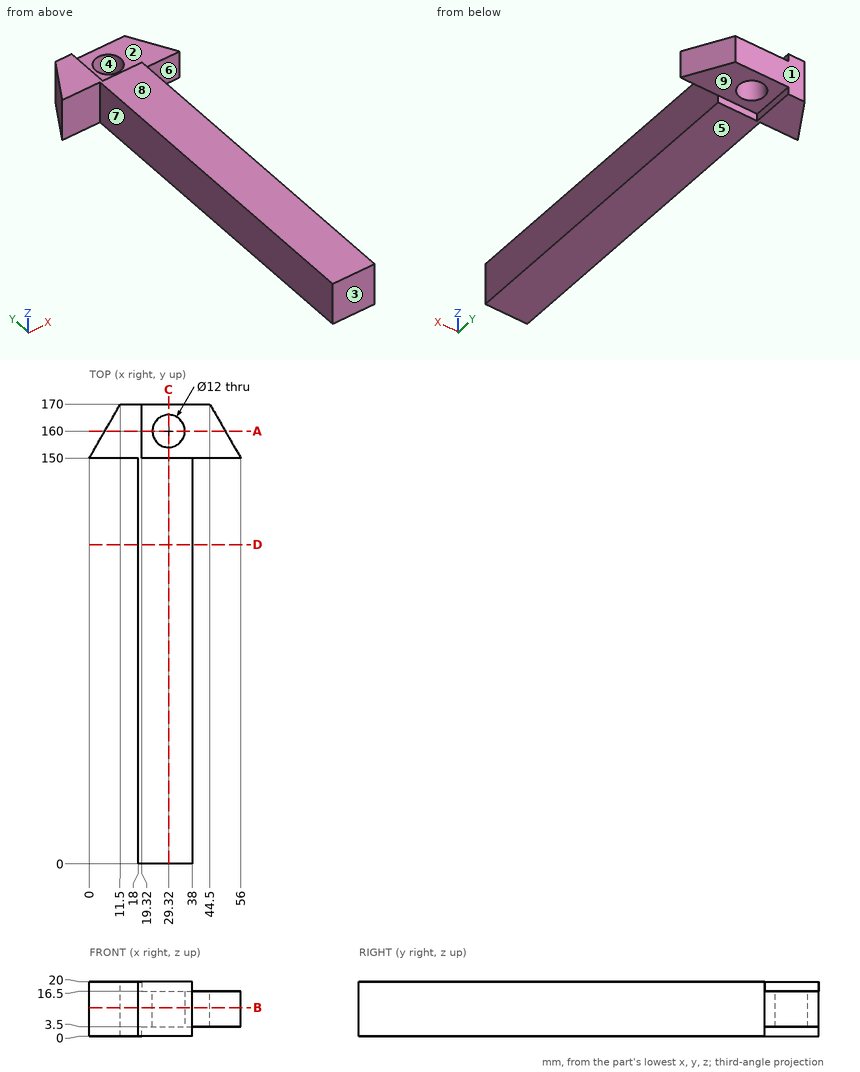
The drawing under review shows one solid part. Ordinate dimensions are in mm from its lowest x, y, z. A direction names the side the tool comes from. Coordinates: 2 decimals unless noted, no trailing zeros. Order: outer loops, then holes, each group sorted by start corner. A loop starts at its lowest first (then second) coordinate and runs counter-clockwise, first axis right, second up. Notation, with made-up numbers: (-40, -22.5) - (11, -22.5) arc R9 cw to (11, -8.5) - close; hole circle Ø1 at (71, 32). An arc over 180 degrees is marked (long way). Put each result on its own line as item: value.
1) Take a section at A-A, the plane y = 160. Give the boundary of the cut face in (x, z).
Response values:
outline: (5.75, 0) - (19.32, 0) - (19.32, 3.5) - (23.32, 3.5) - (23.32, 16.5) - (19.32, 16.5) - (19.32, 20) - (5.75, 20) - close; (35.32, 3.5) - (50.25, 3.5) - (50.25, 16.5) - (35.32, 16.5) - close
2) Insertion check: P1, Ø10, axis at y = 99.5, z = 18, coming from the +X side; P2, Ø6, axis at x = 28.5, y = 156.5, coming from the +Z side; P3, Ø22, axis at x = 29, y = 163, coming from the -Z side; P4, Ø9, axis at x = 11.5, z = 6.5, coming from the -Y side. Each pin has a flat end and moves straight along its axis. Give the tip position at first contact, or say it passes through.
Response values:
P1: stops at x = 38
P2: stops at z = 16.5
P3: stops at z = 0
P4: stops at y = 150
3) Tool access review of the marked faces 5, 6, 7, 8 and 9: name each direction out of +Z, -Z, +X, -X, +Y, -Y from which nothing blocks a thin tool from reaching the whole face with its end or side.
Response values:
face 5: -Z, +X, -X, +Y, -Y
face 6: +Z, -Z, +X, -Y
face 7: +Z, -Z, -X, -Y
face 8: +Z, +X, -X, +Y, -Y
face 9: -Z, +X, +Y
4) Wall thickness on L1, parallel to Y at x = 29.32, z = 8.75; L2, parallel to Y at x = 41, z = 5; L3, parallel to X at y = 13.5, z = 8.5: over which ranges is each line inside the solid? List them lowest first. Write a range as from..to.
Response values:
L1: y = 0..154, 166..170
L2: y = 150..170
L3: x = 18..38
5) Take a section at D-D, the plane y = 118. Give the boundary of the cut face in (x, z).
Response values:
outline: (18, 0) - (38, 0) - (38, 20) - (18, 20) - close
6) Take a section at B-B, the plane z = 10.5. Give the boundary of the cut face in (x, y).
Response values:
outline: (0, 150) - (18, 150) - (18, 0) - (38, 0) - (38, 150) - (56, 150) - (44.5, 170) - (11.5, 170) - close; hole circle Ø12 at (29.32, 160)
7) The part is to be moulded in two halves that separate along Y. For the marked faces 1, 2, 3 and 4, say which applies: released by +Y, released by -Y, zero draft, split by the parting line, or undercut.
Response values:
face 1: released by +Y
face 2: zero draft
face 3: released by -Y
face 4: undercut
8) Take a section at C-C, the plane x = 29.32. Give the boundary of the cut face in (y, z), and give its area (3 significant figures).
Response values:
outline: (0, 0) - (150, 0) - (150, 3.5) - (154, 3.5) - (154, 16.5) - (150, 16.5) - (150, 20) - (0, 20) - close; (166, 3.5) - (170, 3.5) - (170, 16.5) - (166, 16.5) - close
area: 3,100 mm²
